The drawing under review shows one solid part. Ordinate dimensions are in mm from its lowest x, y, z. Round coordinates to 2 decimals unless told otherwise and drop trailing zeros. Order: outer loops, then holes, each group sorted by start corner. A loop starts at its lowest first (then second) coordinate and runs counter-clockwise, first axis right, second up. Notation, with made-up numbers: (14.5, 70.25) -> (21.5, 70.25) arc R19 cw to (21.5, 83.25) -> close; hole circle Ø2 at (-32, 24.5). An arc over 180 degrees is marked (long way). Use a Markdown table: item, result. Add a question column.
1) Wall thickness on line 1 along Y through (x, z) = (50, 4.25); line 2 along X through (y, z) = (19.5, 21.5) (1 decimal); line 3 along Y through (x, z) = (20, 1.75): over which ranges is each line inside the solid? List them lowest first. Write a range as [from, to].
2) Consider section B-B (x = 68.5). State the section outline as (y, z) points, plus the area to 3 significant figures.
3) Consider section C-C (y = 33). State the section outline as (x, z) points (1 decimal).
4) Consider section A-A (z = 3.75). State the section outline as (x, y) points, plus the area to 3 significant figures.
5) Clearance check with flat-ended pins moving along their axes: P1, Ø6, axis at x = 20.5, z = 5.5, coming from the +Y side; P2, Ø6, axis at x = 40, z = 9, coming from the +Y side; P3, Ø12, axis at x = 79.5, z = 20, coming from the +Y side. State where each tip first meets the part, or that it passes through.
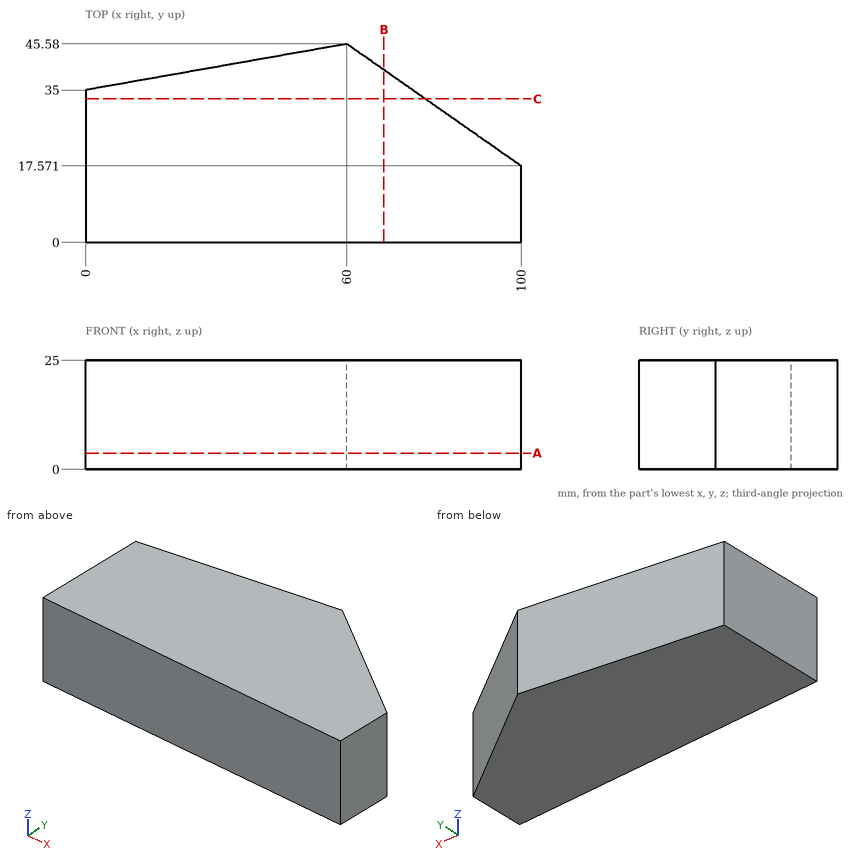
Results list:
| question | item | result |
|---|---|---|
| 1 | line 1 | [0, 43.82] |
| 1 | line 2 | [0, 97.2] |
| 1 | line 3 | [0, 38.53] |
| 2 | outline | (0, 0) -> (39.63, 0) -> (39.63, 25) -> (0, 25) -> close |
| 2 | area | 991 mm2 |
| 3 | outline | (0, 0) -> (78, 0) -> (78, 25) -> (0, 25) -> close |
| 4 | outline | (0, 0) -> (100, 0) -> (100, 17.57) -> (60, 45.58) -> (0, 35) -> close |
| 4 | area | 3,680 mm2 |
| 5 | P1 | y = 39.14 |
| 5 | P2 | y = 42.58 |
| 5 | P3 | y = 36.13 |
